from build123d import *

# Parameters (mm, degrees)
SKETCH_1_W          = 196
SKETCH_1_H          = 221
SKETCH_1_W_2        = 169
SKETCH_1_H_2        = 60
SKETCH_1_W_3        = 149
SKETCH_1_H_3        = 75
SKETCH_1_H_4        = 17
SKETCH_1_W_4        = 159
SKETCH_1_H_5        = 3.5
EXTRUDE_1_DEPTH     = 1.5
SKETCH_5_W          = 7
SKETCH_5_H          = 16
SKETCH_5_H_2        = 15
EXTRUDE_9_DEPTH     = 10
CUT_EXTRUDE_2_DEPTH = 1.4
SKETCH_7_W          = 4
SKETCH_7_H          = 20
EXTRUDE_10_DEPTH    = 75
SKETCH_8_R          = 2.5
CUT_EXTRUDE_3_DEPTH = 185
EXTRUDE_11_DEPTH    = 20


with BuildPart() as part:
    # 草图1 → 凸台-拉伸1 (new body)
    with BuildSketch(Plane(origin=(0, 0, 0), x_dir=(1, 0, 0), z_dir=(0, 1, 0))):
        with Locations((98, 110.5)):
            Rectangle(SKETCH_1_W, SKETCH_1_H)
        with Locations((98, 50)):
            Rectangle(SKETCH_1_W_2, SKETCH_1_H_2, mode=Mode.SUBTRACT)
        with Locations((98, 132.5)):
            Rectangle(SKETCH_1_W_3, SKETCH_1_H_3, mode=Mode.SUBTRACT)
        with Locations((98, 194.5)):
            Rectangle(SKETCH_1_W_3, SKETCH_1_H_4, mode=Mode.SUBTRACT)
        with Locations((106.5, 216.25)):
            Rectangle(SKETCH_1_W_4, SKETCH_1_H_5, mode=Mode.SUBTRACT)
    extrude(amount=EXTRUDE_1_DEPTH)

    # 草图5 → 凸台-拉伸9 (add)
    with BuildSketch(Plane(origin=(0, 0, 0), x_dir=(1, 0, 0), z_dir=(0, 1, 0))):
        Polygon((3, 218), (193, 218), (193, 3), (171.5, 3), (171.5, 20), (178.5, 20), (178.5, 6), (190.27234206, 6), (190.27234206, 213.5), (6.00234206, 213.5), (6.00234206, 6), (17.473925125, 6), (17.473925125, 20), (24.5, 20), (24.5, 3), (3, 3), align=None)
        with Locations((21, 178)):
            Rectangle(SKETCH_5_W, SKETCH_5_H)
        with Locations((175, 178)):
            Rectangle(SKETCH_5_W, SKETCH_5_H)
        with Locations((175, 87.5)):
            Rectangle(SKETCH_5_W, SKETCH_5_H_2)
        with Locations((21, 87.5)):
            Rectangle(SKETCH_5_W, SKETCH_5_H_2)
    extrude(amount=EXTRUDE_9_DEPTH)

    # 草图6 → 切除-拉伸2 (cut)
    with BuildSketch(Plane(origin=(0, 0, 0), x_dir=(1, 0, 0), z_dir=(0, 1, 0))):
        Polygon((27, 217.586317154), (27, 218), (186, 218), (186, 215), (27, 215), align=None)
    extrude(amount=CUT_EXTRUDE_2_DEPTH, mode=Mode.SUBTRACT)

    # 草图7 → 凸台-拉伸10 (add)
    with BuildSketch(Plane(origin=(0, 0, 0), x_dir=(1, 0, 0), z_dir=(0, 1, 0))):
        Polygon((175.5, 132.5), (175.5, 142.5), (171.5, 142.5), (171.5, 122.5), (175.5, 122.5), align=None)
        with Locations((22.5, 132.5)):
            Rectangle(SKETCH_7_W, SKETCH_7_H)
    extrude(amount=EXTRUDE_10_DEPTH)

    # 草图8 → 切除-拉伸3 (cut)
    with BuildSketch(Plane(origin=(175.5, 0, 0), x_dir=(0, 0, -1), z_dir=(1, 0, 0))):
        with Locations((132.5, 66.5)):
            Circle(SKETCH_8_R)
        with Locations((132.5, 54.5)):
            Circle(SKETCH_8_R)
        with Locations((132.5, 23.5)):
            Circle(SKETCH_8_R)
    extrude(amount=-CUT_EXTRUDE_3_DEPTH, mode=Mode.SUBTRACT)

    # 草图10 → 凸台-拉伸11 (add)
    with BuildSketch(Plane(origin=(0, 0, -142.5), x_dir=(-1, 0, 0), z_dir=(0, 0, -1))):
        Polygon((-189.5, 1.5), (-175.5, 1.5), (-175.5, 16.5), align=None)
        Polygon((-20.5, 1.5), (-6.5, 1.5), (-20.5, 16.5), align=None)
    extrude(amount=-EXTRUDE_11_DEPTH)


solid = part.part
Work out the finished part from the listing and answer in its coordinate system (mm). A direction names the side the tool comes from. Give positions to 0.01 mm unless a question says otherwise; leave off trailing zeros. Loops run counter-clockwise (first coordinate to the right, second up) from the corner with the lowest first, then second, coordinate; pieces in that order, holes last. Notation, with made-up numbers: (80, 30) -> (89, 30) arc R10 cw to (89, 46) -> close; hole circle Ø2 at (43.25, 19.25). An arc over 180 degrees is marked (long way). Use a Markdown table: item, result. Add a question column.
1) The part is cut by section D-D, the plane y = 54.5. Determine the outline of the cut face in (x, z), plus the area to 3 significant figures.
2) Each of these flat-tipped pins is pushed along its axis until it touches: P1, Ø20, axis at x = 17, y = 33, coming from the -Z side; P2, Ø2.5, axis at y = 4, z = -181.5, coming from the -X side; P3, Ø11, axis at x = 94.5, y = 2.5, coming from the +Z side; P4, Ø5.5, axis at x = 19.5, y = 24, coming from the +Z side. Where does it stop, or does it pass through?
3) For a pull along X with two mould halves and no side action, classify faces 1 (the flat face through (175, 10, -88)), 2 (the flat face through (20.5, 45, -132)), 3 (the flat face through (178.5, 6, -87)) as +X half, -X half, draft (parallel to the pull), parting line (faces both ways), or undercut.
4) The part is cut by section B-B, the plane z = -197.5. Determine the outline of the cut face in (x, y), plus the area to 3 significant figures.
5) Which of the six approach directions +Z, -Z, +X, -X, +Y, -Y give full straight-line access (tool end or side, diameter ignored) to faces 4 (the flat face through (97, 0, -87)), 5 (the flat face through (98, 1, -20)), 6 (the flat face through (97, 1.5, -88)), 7 (the flat face through (14, 6, -3)), 8 (the flat face through (99, 6, -213.5))?
6) Consider line 1 along Y through (x, z) = (173.95, -132.5); line 2 along Y through (x, z) = (173, -132); line 3 along Z through (x, y) = (174, 66). Determine where each line is inside the solid, lowest interval first.
7) The part is cut by section A-A, the plane y = 43. Determine the outline of the cut face in (x, z), plus the area to 3 significant figures.
8) The part is cut by section C-C, the plane x = 158. Determine the outline of the cut face in (y, z), plus the area to 3 significant figures.
Reported:
| question | item | result |
|---|---|---|
| 1 | outline | (20.5, -142.5) -> (24.5, -142.5) -> (24.5, -135) -> (20.5, -135) -> close; (20.5, -130) -> (24.5, -130) -> (24.5, -122.5) -> (20.5, -122.5) -> close; (171.5, -142.5) -> (175.5, -142.5) -> (175.5, -135) -> (171.5, -135) -> close; (171.5, -130) -> (175.5, -130) -> (175.5, -122.5) -> (171.5, -122.5) -> close |
| 1 | area | 120 mm^2 |
| 2 | P1 | stops at z = -142.5 |
| 2 | P2 | stops at x = 3 |
| 2 | P3 | stops at z = 0 |
| 2 | P4 | stops at z = -122.5 |
| 3 | face 1 | draft |
| 3 | face 2 | -X half |
| 3 | face 3 | undercut |
| 4 | outline | (0, 0) -> (23.5, 0) -> (23.5, 1.5) -> (6, 1.5) -> (6, 10) -> (3, 10) -> (3, 1.5) -> (0, 1.5) -> close; (172.5, 0) -> (196, 0) -> (196, 1.5) -> (193, 1.5) -> (193, 10) -> (190.27, 10) -> (190.27, 1.5) -> (172.5, 1.5) -> close |
| 4 | area | 119 mm^2 |
| 5 | face 4 | +Z, -Z, +X, -X, -Y |
| 5 | face 5 | +Y, -Y |
| 5 | face 6 | +Z, +Y |
| 5 | face 7 | +Z, +X, -X, +Y |
| 5 | face 8 | +Y |
| 6 | line 1 | y = 0 to 21, 26 to 52, 57 to 64, 69 to 75 |
| 6 | line 2 | y = 0 to 21.05, 25.95 to 52.05, 56.95 to 64.05, 68.95 to 75 |
| 6 | line 3 | z = -142.5 to -134.95, -130.05 to -122.5 |
| 7 | outline | (20.5, -142.5) -> (24.5, -142.5) -> (24.5, -122.5) -> (20.5, -122.5) -> close; (171.5, -142.5) -> (175.5, -142.5) -> (175.5, -122.5) -> (171.5, -122.5) -> close |
| 7 | area | 160 mm^2 |
| 8 | outline | (0, -221) -> (1.5, -221) -> (1.5, -218) -> (10, -218) -> (10, -213.5) -> (1.5, -213.5) -> (1.5, -203) -> (0, -203) -> (0, -215) -> (1.4, -215) -> (1.4, -218) -> (0, -218) -> close; (0, -186) -> (1.5, -186) -> (1.5, -170) -> (0, -170) -> close; (0, -95) -> (1.5, -95) -> (1.5, -80) -> (0, -80) -> close; (0, -20) -> (1.5, -20) -> (1.5, 0) -> (0, 0) -> close |
| 8 | area | 138 mm^2 |
